```python
from build123d import *

# Parameters (mm, degrees)
F0_R     = 6.985
F0_R_2   = 2.38125
F0_R_3   = 1.5748
F1_DEPTH = 3.175
F2_DEPTH = 34.9758
F3_DEPTH = 7.0612


with BuildPart() as f1:
    # F0 (on Top) → F1 (new body)
    with BuildSketch(Plane.XY):
        Circle(F0_R)
        Circle(F0_R_2, mode=Mode.SUBTRACT)
        with Locations((0, 4.826)):
            Circle(F0_R_3, mode=Mode.SUBTRACT)
        with Locations((0, 4.826)):
            Circle(F0_R_3)
    extrude(amount=F1_DEPTH)

    # F0 (on Top) → F2 (join)
    with BuildSketch(Plane.XY):
        Circle(F0_R_2)
    extrude(amount=F2_DEPTH)

    # F0 (on Top) → F3 (join)
    with BuildSketch(Plane.XY):
        with Locations((0, 4.826)):
            Circle(F0_R_3)
    extrude(amount=-F3_DEPTH)


solid = f1.part
```
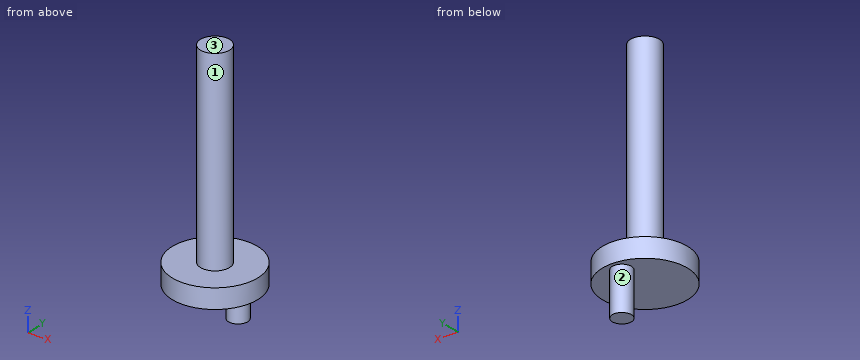
Build history of the part. All positions in model axes, mm. Face numbers are marked on the shaded views. A direction names the side the tool comes from. Round coordinates to 2 decimals unless told otherwise and drop trailing zeros. Loops run counter-clockwise (first coordinate to the right, second up) from the corner with the lowest first, then second, coordinate; pieces in that order, holes last. Notation, with made-up numbers: M -7.75,58.5 L 46.25,58.5 A17 cw 46.25,77.5 Z; hole C 85.5,88 d10. An arc over 180 degrees is marked long. Answer as CSV lines item,"result".
1. Cut at A-A on x = 0. Write the cut outline in (y, z) (3 decimals), then the cut area to 3 significant figures.
Resolved:
outline,"M -6.985,0 L 3.251,0 L 3.251,-7.061 L 6.401,-7.061 L 6.401,0 L 6.985,0 L 6.985,3.175 L 2.381,3.175 L 2.381,34.976 L -2.381,34.976 L -2.381,3.175 L -6.985,3.175 Z"
area,"218 mm²"
2. Flat gauge pins, fed straight in: P1, Ø4, axis at x = 5.5, y = -3, coming from the +Z side (3 decimals); P2, Ø4, axis at x = -1.5, y = -2.5, coming from the +Z side; P3, Ø3, axis at y = -1, z = 7.5, coming from the +X side; P4, Ø8, axis at y = 5.5, z = 21, coming from the +X side. Where does each tip first touch, or does it go through?
Resolved:
P1,"stops at z = 3.175"
P2,"stops at z = 34.98"
P3,"stops at x = 2.38"
P4,"stops at x = 1.85"
3. Wall check: probe 1 along Z at (x, y) = (1.75, 2.75) (3 decimals); probe 2 along Y at (x, z) = (0, 31.5); probe 3 along Z at (x, y) = (0.75, -1.75). Give the ranges that are in metal, low to high. Write a range as [from, to].
Resolved:
probe 1,"z = [0, 3.175]"
probe 2,"y = [-2.38, 2.38]"
probe 3,"z = [0, 34.98]"
4. 3-axis set-ups, long thin cutter, end or side, ignore diameter. For the marked faces 1, 2 and 3: which of +Z, -Z, +X, -X, +Y, -Y reach the whole face in a straight line?
Resolved:
face 1,"+Z"
face 2,"-Z"
face 3,"+Z, +X, -X, +Y, -Y"
5. Cut at B-B on y = 0. Write the cut outline in (x, z) (3 decimals), then the cut area to 3 significant figures.
Resolved:
outline,"M -6.985,0 L 6.985,0 L 6.985,3.175 L 2.381,3.175 L 2.381,34.976 L -2.381,34.976 L -2.381,3.175 L -6.985,3.175 Z"
area,"196 mm²"
6. Cut at C-C on z = 1. Write the cut outline in (x, y) (3 decimals).
Resolved:
outline,"C 0,0 d13.97"
7. Cut at D-D on y = -2. Write the cut outline in (x, z) (3 decimals), then the cut area to 3 significant figures.
Resolved:
outline,"M -6.693,0 L 6.693,0 L 6.693,3.175 L 1.292,3.175 L 1.292,34.976 L -1.292,34.976 L -1.292,3.175 L -6.693,3.175 Z"
area,"125 mm²"
